from build123d import *

# Parameters (mm, degrees)
F0_W      = 117
F0_H      = 77
F1_DEPTH  = 3
F3_DEPTH  = 10
F4_W      = 71
F4_H      = 3
F5_DEPTH  = 3
F6_W      = 111
F6_H      = 3
F7_DEPTH  = 3
F8_W      = 111
F8_H      = 3
F9_DEPTH  = 3
F10_W     = 7.5
F10_H     = 40
F11_DEPTH = 3.5
F13_DEPTH = 40
F14_DEPTH = 40


with BuildPart() as f1:
    # F0 (on Top) → F1 (new body)
    with BuildSketch(Plane.XY):
        with Locations((58.5, 38.5)):
            Rectangle(F0_W, F0_H)
    extrude(amount=F1_DEPTH)

    # F2 (on face) → F3 (join)
    with BuildSketch(Plane.XY.offset(3)):
        Polygon((117, 0), (117, 3), (3, 3), (3, 74), (117, 74), (117, 77), (0, 77), (0, 0), align=None)
    extrude(amount=F3_DEPTH)

    # F4 (on face) → F5 (join)
    with BuildSketch(Plane.YZ.offset(3)):
        with Locations((38.5, 11.5)):
            Rectangle(F4_W, F4_H)
    extrude(amount=F5_DEPTH)

    # F6 (on face) → F7 (join)
    with BuildSketch(Plane(origin=(0, 3, 0), x_dir=(-1, 0, 0), z_dir=(0, 1, 0))):
        with Locations((-61.5, 11.5)):
            Rectangle(F6_W, F6_H)
    extrude(amount=F7_DEPTH)

    # F8 (on face) → F9 (join)
    with BuildSketch(Plane.XZ.offset(-74)):
        with Locations((61.5, 11.5)):
            Rectangle(F8_W, F8_H)
    extrude(amount=F9_DEPTH)

    # F10 (on face) → F11 (join)
    with BuildSketch(Plane(origin=(0, 0, 0), x_dir=(1, 0, 0), z_dir=(0, 0, -1))):
        with Locations((12.25, -57)):
            Rectangle(F10_W, F10_H)
    extrude(amount=F11_DEPTH)

    # F12 (on face) → F13 (cut)
    with BuildSketch(Plane(origin=(0, 77, 0), x_dir=(-1, 0, 0), z_dir=(0, 1, 0))):
        Polygon((-16, 0), (-16, -3.5), (-15, 0), align=None)
    extrude(amount=-F13_DEPTH, mode=Mode.SUBTRACT)

    # F12 (on face) → F14 (cut)
    with BuildSketch(Plane(origin=(0, 77, 0), x_dir=(-1, 0, 0), z_dir=(0, 1, 0))):
        Polygon((-9.5, 0), (-8.5, -3.5), (-8.5, 0), align=None)
    extrude(amount=-F14_DEPTH, mode=Mode.SUBTRACT)


solid = f1.part
Work out the finished part from the listing and answer in its coordinate system (mm). A direction names the side the tool comes from. Give positions to 0.01 mm unless a question says otherwise; leave off trailing zeros. Loops run counter-clockwise (first coordinate to the right, second up) from the corner with the lowest first, then second, coordinate; pieces in that order, holes last. Notation, with made-up numbers: (-24, -33) -> (-16, -33) arc R19 cw to (-16, -22) -> close; hole circle Ø5 at (1, -7). An arc over 180 degrees is marked (long way). Use a Markdown table: item, result. Add a question column.
1) For a pull along Z with two mould halves and no side action, classify faces 1 (the flat face through (3, 38, 6)), 2 (the flat face through (12, 57, -3.5)), 3 (the flat face through (6, 38, 12)) as +Z half, -Z half, draft (parallel to the pull), parting line (faces both ways), or undercut.
2) Consider line 1 along Y through (x, z) = (63, 8.25); line 2 along Y through (x, z) = (38, 12.25); line 3 along Z through (x, y) = (77, 51). Determine where each line is inside the solid, lowest interval first.
3) Each of these flat-tipped pins is pushed along its axis until it touches: P1, Ø4, axis at y = 53.5, z = 7.5, coming from the +X side; P2, Ø4, axis at x = 31.5, y = 35.5, coming from the -Z side; P3, Ø5.5, axis at y = 51.5, z = 7.5, coming from the +X side. Where does it stop, or does it pass through?
4) The part is cut by section C-C, the plane z = 11.5. Determine the outline of the cut face in (x, y).
5) The part is cut by section D-D, the plane y = 26.5. Determine the outline of the cut face in (x, z), plus the area to 3 significant figures.
6) The part is cut by section A-A, the plane y = 64. Determine the outline of the cut face in (x, z).
7) The part is cut by section B-B, the plane x = 71. Determine the outline of the cut face in (y, z).
8) Which of the six approach directions +Z, -Z, +X, -X, +Y, -Y give full straight-line access (tool end or side, diameter ignored) to faces 4 (the flat face through (15.507, 57.28, -1.774)), 5 (the flat face through (50, 4, 13)), 6 (the flat face through (43, 73, 10)), 7 (the flat face through (62, 6, 12)), 8 (the flat face through (12, 37, -2))?
Reported:
| question | item | result |
|---|---|---|
| 1 | face 1 | undercut |
| 1 | face 2 | -Z half |
| 1 | face 3 | draft |
| 2 | line 1 | y = 0 to 3, 74 to 77 |
| 2 | line 2 | y = 0 to 6, 71 to 77 |
| 2 | line 3 | z = 0 to 3 |
| 3 | P1 | stops at x = 3 |
| 3 | P2 | stops at z = 0 |
| 3 | P3 | stops at x = 6 |
| 4 | outline | (0, 0) -> (117, 0) -> (117, 6) -> (6, 6) -> (6, 71) -> (117, 71) -> (117, 77) -> (0, 77) -> close |
| 5 | outline | (0, 0) -> (117, 0) -> (117, 3) -> (3, 3) -> (3, 10) -> (6, 10) -> (6, 13) -> (0, 13) -> close |
| 5 | area | 390 mm^2 |
| 6 | outline | (0, 0) -> (9.5, 0) -> (8.5, -3.5) -> (16, -3.5) -> (15, 0) -> (117, 0) -> (117, 3) -> (3, 3) -> (3, 10) -> (6, 10) -> (6, 13) -> (0, 13) -> close |
| 7 | outline | (0, 0) -> (77, 0) -> (77, 13) -> (71, 13) -> (71, 10) -> (74, 10) -> (74, 3) -> (3, 3) -> (3, 10) -> (6, 10) -> (6, 13) -> (0, 13) -> close |
| 8 | face 4 | +X, +Y, -Y |
| 8 | face 5 | +Z, +X, -X, +Y, -Y |
| 8 | face 6 | +X |
| 8 | face 7 | +Z, +X |
| 8 | face 8 | -Z, +X, -X, -Y |
